Model file for the job. Use its own axes, mm. A direction names the side the tool comes from. Round coordinates to 2 decimals unless told otherwise and drop trailing zeros. Order: outer loops, then holes, each group sorted by start corner. A loop starts at its lowest first (then second) coordinate and runs counter-clockwise, first axis right, second up. Notation, with made-up numbers: (-9.75, -34) -> (49.25, -34) arc R25 ccw to (49.25, -11) -> close; hole circle Ø7 at (-29, 13.5). An arc over 180 degrees is marked (long way). Put each result on its own line as item: value. Start each with the question number.
Q1. Cut at A-A, the plane z = 2.75. List the corners of the cut face in (x, y), and give its area (3 significant figures).
Q2. 3-axis set-ups, long thin cutter, end or side, ignore diameter. For faces 4 (the face through (-0.4, -0.9, -4.2)), 5 (the face through (3.405, -0.444, 2.74)): which of +Z, -Z, +X, -X, +Y, -Y reach the whole face in a straight line?
Q3. Cut at C-C, the plane z = -1. List the corners of the cut face in (x, y), and give its area (3 significant figures).
Q4. Pull direction X, two halves, no side cores. Call faces 1 (the face through (-4.3, -0.4, 3.1)), 2 (the face through (-0.4, 0, -4.2)), 3 (the face through (-4.538, -0.444, 4.496)): released by +X, released by -X, zero draft, split by the parting line, or undercut.
Q5. Cut at D-D, the plane x = -0.75. List the corners of the cut face in (y, z), and give its area (3 significant figures).
Q6. Probe L1, parallel to X at y = -0.05, z = 0; L2, parallel to X at y = -0.1, z = -0.75; L3, parallel to Z at x = 0, y = -0.25. List the from-to ranges inside material, lowest first.
Q7. Cut at B-B, the plane y = -0.2. List the corners of the cut face in (x, z).
from build123d import *
from build123d import SkipClean  # not in build123d's __all__

# Parameters (mm, degrees)
F1_DEPTH = 0.9


with BuildPart() as f1:
    # F0 (on Front) → F1 (new body)
    with BuildSketch(Plane.XZ):
        with BuildLine():
            ThreePointArc((-3.6648012211, 1.333878559), (-3.4047554287, 2.7601313999), (-3.6315648982, 4.1920456588))
            ThreePointArc((-3.6315648982, 4.1920456588), (-4.5505468427, 4.4869465177), (-4.562494352, 3.5218809304))
            ThreePointArc((-4.562494352, 3.5218809304), (-4.2983800559, 3.0982301484), (-4.3837176879, 2.6063421173))
            ThreePointArc((-4.3837176879, 2.6063421173), (-4.4329642903, -2.5216715886), (0, -5.1))
            Line((0, -5.1), (0, -3.9))
            ThreePointArc((0, -3.9), (-3.1946929727, -2.2369481018), (-3.6648012211, 1.333878559))
        make_face()
    extrude(amount=F1_DEPTH)

    # F2: F1 across plane


with BuildPart() as f1_1:
    add(f1.part, clean=False)
    with SkipClean():  # cleaning this boolean's faces spoils the solid; the shape is the same uncleaned
        add(f1.part.mirror(Plane.YZ), clean=False)


solid = f1_1.part
Ans:
1. outline: (-4.32, -0.9) -> (-3.4, -0.9) -> (-3.4, 0) -> (-4.32, 0) -> close; (3.4, -0.9) -> (4.32, -0.9) -> (4.32, 0) -> (3.4, 0) -> close
1. area: 1.65 mm^2
2. face 4: +Z, -Z, +X, -X, -Y
2. face 5: +Y, -Y
3. outline: (-5, -0.9) -> (-3.77, -0.9) -> (-3.77, 0) -> (-5, 0) -> close; (3.77, -0.9) -> (5, -0.9) -> (5, 0) -> (3.77, 0) -> close
3. area: 2.22 mm^2
4. face 1: released by -X
4. face 2: zero draft
4. face 3: undercut
5. outline: (-0.9, -5.04) -> (0, -5.04) -> (0, -3.83) -> (-0.9, -3.83) -> close
5. area: 1.10 mm^2
6. L1: x = -5.1 to -3.9, 3.9 to 5.1
6. L2: x = -5.04 to -3.83, 3.83 to 5.04
6. L3: z = -5.1 to -3.9
7. outline: (-4.56, 3.52) arc R0.7 cw to (-4.38, 2.61) arc R5.1 ccw (long way) to (4.38, 2.61) arc R0.7 cw to (4.56, 3.52) arc R0.6 ccw (long way) to (3.63, 4.19) arc R4.32 ccw to (3.66, 1.33) arc R3.9 cw (long way) to (-3.66, 1.33) arc R4.32 ccw to (-3.63, 4.19) arc R0.6 ccw (long way) to start
